```python
from build123d import *

# Parameters (mm, degrees)
SKETCH_1_R      = 3
SKETCH_4_R      = 2.5
EXTRUDE_1_DEPTH = 11.25


with BuildPart() as part:
    # Sweep 1: sweep along a path in Sketch 2
    with BuildLine(Plane.XY) as sweep_1_path:
        Line((0, 0), (0, -30))
        Line((0, -30), (60, -30))
        Line((60, -30), (60, 0))
    # Sketch 1 → Sweep 1 (sweep)
    with BuildSketch(Plane(origin=(0, 0, 0), x_dir=(1, 0, 0), z_dir=(0, 1, 0))):
        Circle(SKETCH_1_R)
    sweep(path=sweep_1_path.line, transition=Transition.RIGHT)

    # Sketch 4 → Extrude 1 (add)
    with BuildSketch(Plane(origin=(30, -30.150206029, 1.8381e-05), x_dir=(1, 0, 0), z_dir=(0, 1, 0))):
        with Locations(Location((0, 0, 0), (0, 0, 270))):
            Circle(SKETCH_4_R)
    extrude(amount=-EXTRUDE_1_DEPTH)


solid = part.part
```
Model file for the job. Use its own axes, mm. A direction names the side the tool comes from. Round coordinates to 2 decimals unless told otherwise and drop trailing zeros. Write each loop counter-clockwise with the first axis right and the second up, starting at its lowest first coordinate (ties: lowest second). Pieces come first, ordered by that corner, then holes. Notation, with made-up numbers: (-25, 36.25) - (26, 36.25) arc R13 ccw to (26, 43.25) - close; hole circle Ø3 at (-8, 55). An arc over 180 degrees is marked (long way). One line per item, written item: value.
(1) Cut at B-B, the plane y = -4. Give the cut face in (x, z).
Values follow:
outline: circle Ø6 at (0, 0); circle Ø6 at (60, 0)
(2) Cut at C-C, the plane x = 51.5. Give the cut face in (y, z), plus the area to 3 significant figures.
Values follow:
outline: circle Ø6 at (-30, 0)
area: 28.3 mm²
(3) Wall check: probe 1 along X at (y, z) = (-16, -0.25); probe 2 along X at (y, z) = (-10, -2); probe 3 along Y at (x, z) = (54, 0). Give the ranges that are in metal, low to high.
Values follow:
probe 1: x = -2.99 to 2.99, 57.01 to 62.99
probe 2: x = -2.24 to 2.24, 57.76 to 62.24
probe 3: y = -33 to -27
(4) Cut at A-A, the plane z = 0. Give the cut face in (x, y), plus the area to 3 significant figures.
Values follow:
outline: (-3, -33) - (27.5, -33) - (27.5, -41.4) - (32.5, -41.4) - (32.5, -33) - (63, -33) - (63, 0) - (57, 0) - (57, -27) - (3, -27) - (3, 0) - (-3, 0) - close
area: 762 mm²
(5) Two-plate mould, pull along X, no slides. Class faces 1 (the cylindrical face through (30.751, -36.461, 2.385)), 2 (the cylindrical face through (63, -16, 0)), 3 (the flat face through (60, 0, 0)): pulls with the +X half, pulls with the -X half, needs draft (parallel to the pull), parting line crosses it, or undercut.
Values follow:
face 1: parting line crosses it
face 2: undercut
face 3: needs draft
(6) 3-axis set-ups, long thin cutter, end or side, ignore diameter. For faces 4 (the cylindrical face through (-3, -17, 0)), 5 (the flat face through (30, -41.4, 0)), 6 (the cylindrical face through (30.46, -30.65, -2.93)): which of +Z, -Z, +X, -X, +Y, -Y reach the whole face in a straight line?
Values follow:
face 4: +Y
face 5: +Z, -Z, +X, -X, -Y
face 6: none
(7) Cut at D-D, the plane y = -30. Give the cut face in (x, z).
Values follow:
outline: (0, -3) - (60, -3) arc R3 ccw to (60, 3) - (0, 3) arc R3 ccw to start
(8) Drop flat-ended pins along their axis: P1, Ø1, axis at x = 26, z = -1.5, coming from the -Y side; P2, Ø2, axis at y = -8.5, z = -0.5, coming from the +X side; P3, Ø1, axis at x = 22.5, z = -1.5, coming from the +Y side. Give the stop position or say it passes through.
Values follow:
P1: stops at y = -32.83
P2: stops at x = 63
P3: stops at y = -27.17
